from build123d import *

# Parameters (mm, degrees)
SKETCH1_R           = 2.286
SKETCH1_R_2         = 2.667
BOSS_EXTRUDE1_DEPTH = 10.16
SKETCH7_R           = 3.6195
SKETCH7_R_2         = 4.6355
CUT_EXTRUDE1_DEPTH  = 4.064
SKETCH3_R           = 1.397
CUT_EXTRUDE2_DEPTH  = 1.016
SKETCH8_R           = 1.397
CUT_EXTRUDE3_DEPTH  = 1.016
CUT_EXTRUDE4_START  = -1.016
SKETCH9_R           = 1.397
CUT_EXTRUDE4_DEPTH  = 1.016


with BuildPart() as part:
    # Sketch1 → Boss-Extrude1 (new body)
    with BuildSketch(Plane.XY):
        Polygon((0, 57.15), (12.7, 57.15), (12.7, 67.31), (25.4, 67.31), (25.4, 57.15), (38.1, 57.15), (38.1, 0), (0, 0), align=None)
        with Locations((5.08, 7.62)):
            Circle(SKETCH1_R, mode=Mode.SUBTRACT)
        with Locations((5.08, 30.48)):
            Circle(SKETCH1_R, mode=Mode.SUBTRACT)
        with Locations((26.67, 15.24)):
            Circle(SKETCH1_R_2, mode=Mode.SUBTRACT)
        with Locations((22.86, 30.48)):
            Circle(SKETCH1_R, mode=Mode.SUBTRACT)
    extrude(amount=BOSS_EXTRUDE1_DEPTH)

    # Sketch7 → Cut-Extrude1 (cut)
    with BuildSketch(Plane.XY.offset(10.16)):
        with Locations((5.08, 30.48)):
            Circle(SKETCH7_R)
        with Locations((22.86, 30.48)):
            Circle(SKETCH7_R)
        with Locations((5.08, 7.62)):
            Circle(SKETCH7_R)
        with Locations((26.67, 15.24)):
            Circle(SKETCH7_R_2)
    extrude(amount=-CUT_EXTRUDE1_DEPTH, mode=Mode.SUBTRACT)

    # Sketch3 → Cut-Extrude2 (cut)
    with BuildSketch(Plane(origin=(0, 0, 10.16), x_dir=(-1, 0, 0), z_dir=(0, 0, -1))):
        with Locations((-19.05, 62.23)):
            Circle(SKETCH3_R)
    extrude(amount=CUT_EXTRUDE2_DEPTH, mode=Mode.SUBTRACT)

    # Sketch8 → Cut-Extrude3 (cut)
    with BuildSketch(Plane(origin=(25.4, 0, 0), x_dir=(0, 0, -1), z_dir=(1, 0, 0))):
        with Locations((-5.08, 62.23)):
            Circle(SKETCH8_R)
    extrude(amount=-CUT_EXTRUDE3_DEPTH, mode=Mode.SUBTRACT)

    # Sketch9 → Cut-Extrude4 (cut)
    with BuildSketch(Plane.ZY.offset(-12.7).offset(CUT_EXTRUDE4_START)):
        with Locations(Location((5.08, 62.23, 0), (0, 0, 180))):
            Circle(SKETCH9_R)
    extrude(amount=CUT_EXTRUDE4_DEPTH, mode=Mode.SUBTRACT)


solid = part.part
Can you work these out from the model? Positions are in its coordinate system, mm. A direction names the side the tool comes from. Coordinates: 2 decimals unless noted, no trailing zeros. Write each loop counter-clockwise with the first axis right and the second up, starting at its lowest first coordinate (ties: lowest second). Pieces come first, ordered by that corner, then holes. Notation, with made-up numbers: (63, 63.25) -> (73, 63.25) arc R4 ccw to (73, 67.25) -> close; hole circle Ø1 at (-6.5, 39). An arc over 180 degrees is marked (long way). Write each question's results on one line, items separated by ' | '. Start each with the question number.
Item 1: If we section it at D-D, the plane x = 22.86: Write out the boundary of the cut face in (y, z), and give its area (3 significant figures).
Item 2: Please list where these lines run through material, in increasing order: probe 1 along Y at (x, z) = (5.08, 4.25); probe 2 along X at (y, z) = (7.62, 3.5); probe 3 along X at (y, z) = (30.48, 1.75).
Item 3: Thinking about a two-plate mould opening in X: for faces 1 (the cylindrical face through (18.41, 60.99, 9.66)), 2 (the flat face through (13.716, 62, 5)), 3 (the flat face through (25.4, 63.4, 3.9)), which applies, released by +X, released by -X, zero draft, split by the parting line, or undercut?
Item 4: On a 3-axis mill with a long thin cutter (end or side, diameter ignored), from which of +Z, -Z, +X, -X, +Y, -Y can I reach the whole of each face in a straight line? I mean faces 4 (the cylindrical face through (24.899, 60.866, 5.383)), 5 (the flat face through (5, 28, 6.096)), 6 (the cylindrical face through (13.215, 63.594, 5.383)). Say none if no direction works.
Item 5: If we section it at A-A, the plane y = 30.48: Write out the boundary of the cut face in (x, z).
Item 6: I'm going to push flat-ended pins straight in: P1, Ø5, axis at x = 28, z = 3, coming from the +Y side; P2, Ø2, axis at y = 63, z = 4.5, coming from the -X side; P3, Ø2.5, axis at x = 19.05, y = 62.23, coming from the +Z side. Where does each tip first touch, or does it pass through?
Item 7: If we section it at C-C, the plane y = 15.24: Write out the boundary of the cut face in (x, z).
Item 8: If we section it at B-B, the plane z = 7.5: Write out the boundary of the cut face in (x, y).
Answer block:
1) outline: (0, 0) -> (28.19, 0) -> (28.19, 6.1) -> (26.86, 6.1) -> (26.86, 10.16) -> (17.88, 10.16) -> (17.88, 6.1) -> (12.6, 6.1) -> (12.6, 10.16) -> (0, 10.16) -> close; (32.77, 0) -> (67.31, 0) -> (67.31, 10.16) -> (34.1, 10.16) -> (34.1, 6.1) -> (32.77, 6.1) -> close | area: 605 mm²
2) probe 1: 0 to 5.33, 9.91 to 28.19, 32.77 to 57.15 | probe 2: 0 to 2.79, 7.37 to 38.1 | probe 3: 0 to 2.79, 7.37 to 20.57, 25.15 to 38.1
3) face 1: undercut | face 2: released by -X | face 3: released by +X
4) face 4: +X | face 5: +Z | face 6: -X
5) outline: (0, 0) -> (2.79, 0) -> (2.79, 6.1) -> (1.46, 6.1) -> (1.46, 10.16) -> (0, 10.16) -> close; (7.37, 0) -> (20.57, 0) -> (20.57, 6.1) -> (19.24, 6.1) -> (19.24, 10.16) -> (8.7, 10.16) -> (8.7, 6.1) -> (7.37, 6.1) -> close; (25.15, 0) -> (38.1, 0) -> (38.1, 10.16) -> (26.48, 10.16) -> (26.48, 6.1) -> (25.15, 6.1) -> close
6) P1: y = 57.15 | P2: x = 12.7 | P3: z = 9.14
7) outline: (0, 0) -> (24, 0) -> (24, 6.1) -> (22.03, 6.1) -> (22.03, 10.16) -> (0, 10.16) -> close; (29.34, 0) -> (38.1, 0) -> (38.1, 10.16) -> (31.31, 10.16) -> (31.31, 6.1) -> (29.34, 6.1) -> close
8) outline: (0, 0) -> (38.1, 0) -> (38.1, 57.15) -> (25.4, 57.15) -> (25.4, 67.31) -> (12.7, 67.31) -> (12.7, 57.15) -> (0, 57.15) -> close; hole circle Ø7.24 at (5.08, 7.62); hole circle Ø7.24 at (5.08, 30.48); hole circle Ø7.24 at (22.86, 30.48); hole circle Ø9.27 at (26.67, 15.24)
